Could you check a few things on this model? Use its own coordinates, in mm. A direction names the side the tool comes from. Coordinates: 2 decimals unless noted, no trailing zeros. Order: outer loops, then holes, each group sorted by start corner. A loop starts at its lowest first (then second) coordinate and runs counter-clockwise, first axis right, second up. Notation, with made-up numbers: (5, -16.5) - (14, -16.5) arc R24 ccw to (14, -3.5) - close; hole circle Ø6 at (9.5, 16). An arc over 180 degrees is marked (long way). Answer as CSV lines item,"result". Start each with the question number.
1. I want a section at B-B, the plane z = 6.25. List the corners of the cut face in (x, y) for me.
2. Thinking about a two-plate mould opening in Z: for faces 1 (the face through (-15, 3, 2.966)), 2 (the face through (8.695, 3, 0)), 3 (the face through (17.505, 0.751, -9.597)), which applies, released by +Z, released by -Z, zero draft, split by the parting line, or undercut?
3. I want a section at A-A, the plane y = 2.55. List the corners of the cut face in (x, z) for me.
4. I want a section at C-C, the plane x = 65. List the corners of the cut face in (y, z) for me (3 decimals).
5. I need wall thicknesses on probe 1 along X at (y, z) = (0.5, 5); probe 2 along Y at (x, z) = (8, 5.5); probe 3 along X at (y, z) = (4.3, -1.25). Which ranges of each line are inside material? Lowest first, please.
6. For pin 1 (0.8 mm diameter, centred on y = 3, z = 1.5, fed in from +X); pin 2 (3 mm diameter, centred on x = -15.875, z = 9.525, fed in from -Y); pin 3 (0.5 mm diameter, centred on y = 0.5, z = -5, fed in from +X); pin 4 (1.5 mm diameter, centred on x = 21, y = 1.5, fed in from -Z) (3 decimals), each with a flat end and sliding along its axis, tell me the tip position at first contact or that it passes through.
7. For faces 4 (the face through (-9.508, 3, 1)), 5 (the face through (-8.4, 2.8, -8.1)), 6 (the face through (-1, 4.064, 0)), which set-ups out of +Z, -Z, +X, -X, +Y, -Y let a thin tool reach every point of the face, with its end or its side?
from build123d import *

# Parameters (mm, degrees)
SKETCH1_W             = 38.1
SKETCH1_H             = 25.4
BOSS_EXTRUDE1_DEPTH   = 1.524
F_4_CLEARANCE_HOLE1_D = 3.2639
BOSS_EXTRUDE2_DEPTH   = 2.54
SKETCH2_3_W           = 3.097805831
SKETCH2_3_H           = 5.99739549
SKETCH2_3_W_2         = 4.661851382
BOSS_EXTRUDE3_DEPTH   = 3.175
SKETCH6_R             = 0.635
BOSS_EXTRUDE4_DEPTH   = 76.2


with BuildPart() as part:
    # Sketch1 → Boss-Extrude1 (new body)
    with BuildSketch(Plane(origin=(0, 0, 0), x_dir=(1, 0, 0), z_dir=(0, 1, 0))):
        Rectangle(SKETCH1_W, SKETCH1_H)
    extrude(amount=BOSS_EXTRUDE1_DEPTH)

    # 4 Clearance Hole1 (through all)
    with Locations(Plane(origin=(0, 1.524, 0), x_dir=(1, 0, 0), z_dir=(0, 1, 0))):
        with Locations((-15.875, 9.525), (15.875, 9.525), (15.875, -9.525), (-15.875, -9.525)):
            Hole(F_4_CLEARANCE_HOLE1_D / 2)

    # Sketch2 → Boss-Extrude2 (add)
    with BuildSketch(Plane(origin=(0, 1.524, 0), x_dir=(1, 0, 0), z_dir=(0, 1, 0))):
        Polygon((-9.50810694, -9.112699607), (8.695477597, -9.112699607), (8.695477597, 9.104771495), (-7.397734973, 9.104771495), (-9.50810694, 6.994399527), align=None)
    extrude(amount=BOSS_EXTRUDE2_DEPTH)

    # Sketch2_3 → Boss-Extrude3 (add)
    with BuildSketch(Plane(origin=(0, 1.524, 0), x_dir=(1, 0, 0), z_dir=(0, 1, 0))):
        with Locations((-17.423902916, 0.033144474)):
            Rectangle(SKETCH2_3_W, SKETCH2_3_H)
        with Locations((-13.544074309, 0.033144474)):
            Rectangle(SKETCH2_3_W_2, SKETCH2_3_H)
    extrude(amount=BOSS_EXTRUDE3_DEPTH)

    # Sketch6 → Boss-Extrude4 (add)
    with BuildSketch(Plane(origin=(19.05, 0, 0), x_dir=(0, 0, -1), z_dir=(1, 0, 0))):
        with Locations((0, 0.762)):
            Circle(SKETCH6_R)
    extrude(amount=BOSS_EXTRUDE4_DEPTH)


solid = part.part
Solved:
1,outline,"(-19.05, 0) - (19.05, 0) - (19.05, 1.52) - (8.7, 1.52) - (8.7, 4.06) - (-9.51, 4.06) - (-9.51, 1.52) - (-19.05, 1.52) - close"
2,face 1,"released by +Z"
2,face 2,"zero draft"
2,face 3,"undercut"
3,outline,"(-18.97, -3.03) - (-11.21, -3.03) - (-11.21, 2.97) - (-18.97, 2.97) - close; (-9.51, -6.99) - (-7.4, -9.1) - (8.7, -9.1) - (8.7, 9.11) - (-9.51, 9.11) - close"
4,outline,"circle Ø1.27 at (0.762, 0)"
5,probe 1,"x = -19.05 to 19.05"
5,probe 2,"y = 0 to 4.06"
5,probe 3,"x = -18.97 to -11.21"
6,pin 1,"stops at x = 8.7"
6,pin 2,"passes through"
6,pin 3,"stops at x = 19.05"
6,pin 4,"stops at z = -0.635"
7,face 4,"+Z, -Z, +Y"
7,face 5,"-Z, -X, +Y"
7,face 6,"+Z, -Z, +X, +Y"
